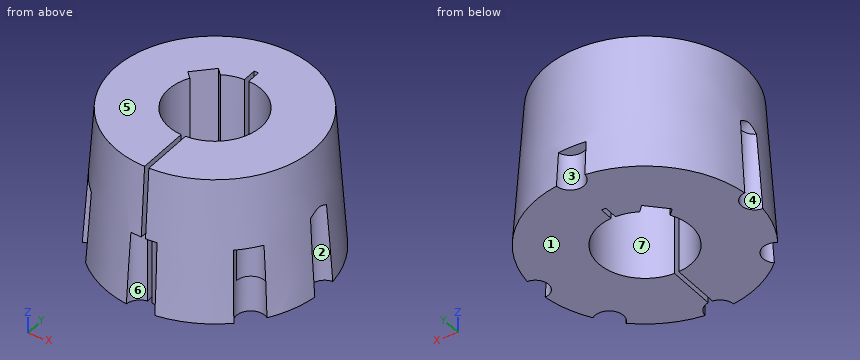
from build123d import *

# Parameters (mm, degrees)
CIRPATTERN1_COUNT       = 2
SKETCH7_R               = 10
CUT_EXTRUDE1_DEPTH      = 25
CIRPATTERN2_COUNT       = 2
CIRPATTERN2_ANGLE       = 130
SKETCH8_R               = 10
CUT_EXTRUDE2_DEPTH      = 50
CIRPATTERN3_COUNT       = 2
CIRPATTERN3_ANGLE       = 50
CUT_EXTRUDE3_DEPTH      = 1022.226122136
CUT_EXTRUDE3_DEPTH_BACK = 1022.226122136
SKETCH9_W               = 3
SKETCH9_H               = 87.216165293
CUT_EXTRUDE4_DEPTH      = 1022.226122136
CUT_EXTRUDE4_DEPTH_BACK = 1022.226122136
SKETCH12_R              = 10
CUT_EXTRUDE6_DEPTH      = 50
CUT_EXTRUDE7_DEPTH      = 1022.226122136
CUT_EXTRUDE7_DEPTH_BACK = 1022.226122136


with BuildPart() as part:
    # Sketch1 → Revolve1 (revolve)
    with BuildSketch(Plane(origin=(0, 0, 0), x_dir=(0, 0, -1), z_dir=(1, 0, 0)), mode=Mode.PRIVATE) as revolve1_sk:
        Polygon((627.254740219, 1014.21395543), (528.454740219, 1007.30518641), (528.454740219, 969.80518641), (532.567237031, 969.80518641), (611.238311694, 969.80518641), (627.254740219, 969.80518641), align=None)
    revolve(revolve1_sk.sketch.rotate(Axis((0, 937.30518641, -528.454740219), (0, 0, -1)), 90), axis=Axis((0, 937.30518641, -528.454740219), (0, 0, -1)))

    # Sketch6 → M20x1.5 Tapped Hole1 (revolve, cut)
    with BuildSketch(Plane(origin=(-76.90876902, 937.30518641, -627.254740219), x_dir=(0, 1, 0), z_dir=(1, 0, 0))):
        Polygon((0, 0), (0, 60.057960726), (9.25, 54.5), (9.25, 0), align=None)
    m20x1_5_tapped_hole1 = revolve(axis=Axis((-76.90876902, 937.30518641, -633.604740219), (0, 0, 1)), mode=Mode.SUBTRACT)

    # CirPattern1: M20x1.5 Tapped Hole1 ×2 about axis
    cirpattern1_axis = Axis((0, 937.30518641, 0), (0, 0, 1))
    for i in range(1, CIRPATTERN1_COUNT):
        add(m20x1_5_tapped_hole1.rotate(cirpattern1_axis, i * 360 / CIRPATTERN1_COUNT), mode=Mode.SUBTRACT)

    # Sketch7 → Cut-Extrude1 (cut)
    with BuildSketch(Plane(origin=(0, 0, -627.254740219), x_dir=(-1, 0, 0), z_dir=(0, 0, -1))):
        with Locations((0, 1014.21395543)):
            Circle(SKETCH7_R)
    cut_extrude1 = extrude(amount=-CUT_EXTRUDE1_DEPTH, mode=Mode.SUBTRACT)

    # CirPattern2: Cut-Extrude1 ×2 about axis
    cirpattern2_axis = Axis((0, 937.30518641, -627.254740219), (0, 0, -1))
    for i in range(1, CIRPATTERN2_COUNT):
        add(cut_extrude1.rotate(cirpattern2_axis, i * CIRPATTERN2_ANGLE / (CIRPATTERN2_COUNT - 1)), mode=Mode.SUBTRACT)

    # Sketch8 → Cut-Extrude2 (cut)
    with BuildSketch(Plane(origin=(0, 0, -627.254740219), x_dir=(-1, 0, 0), z_dir=(0, 0, -1))):
        with Locations((0, 860.39641739)):
            Circle(SKETCH8_R)
    cut_extrude2 = extrude(amount=-CUT_EXTRUDE2_DEPTH, mode=Mode.SUBTRACT)

    # CirPattern3: Cut-Extrude2 ×2 about axis
    cirpattern3_axis = Axis((0, 937.30518641, -627.254740219), (0, 0, -1))
    for i in range(1, CIRPATTERN3_COUNT):
        add(cut_extrude2.rotate(cirpattern3_axis, i * CIRPATTERN3_ANGLE / (CIRPATTERN3_COUNT - 1)), mode=Mode.SUBTRACT)

    # Sketch9 → Cut-Extrude3 (cut, two sides: drawn at the far end of the back side and taken through both)
    with BuildSketch(Plane(origin=(0, 0, -627.254740219), x_dir=(-1, 0, 0), z_dir=(0, 0, -1)).offset(-CUT_EXTRUDE3_DEPTH_BACK)):
        with Locations((0, 893.697103764)):
            Rectangle(SKETCH9_W, SKETCH9_H)
    extrude(amount=CUT_EXTRUDE3_DEPTH + CUT_EXTRUDE3_DEPTH_BACK, mode=Mode.SUBTRACT)

    # Sketch10 → Cut-Extrude4 (cut, two sides: drawn at the far end of the back side and taken through both)
    with BuildSketch(Plane(origin=(0, 0, -627.254740219), x_dir=(-1, 0, 0), z_dir=(0, 0, -1)).offset(-CUT_EXTRUDE4_DEPTH_BACK)):
        Polygon((1.5, 957.30518641), (1.5, 979.639325832), (-1.5, 979.639325832), (-1.5, 957.30518641), (-1.5, 953.730478501), (1.5, 953.730478501), align=None)
    extrude(amount=CUT_EXTRUDE4_DEPTH + CUT_EXTRUDE4_DEPTH_BACK, mode=Mode.SUBTRACT)

    # Sketch12 → Cut-Extrude6 (cut)
    with BuildSketch(Plane(origin=(0, 0, -627.254740219), x_dir=(-1, 0, 0), z_dir=(0, 0, -1))):
        with Locations((-58.915535135, 887.869182608)):
            Circle(SKETCH12_R)
    extrude(amount=-CUT_EXTRUDE6_DEPTH, mode=Mode.SUBTRACT)

    # Sketch13 → Cut-Extrude7 (cut, two sides: drawn at the far end of the back side and taken through both)
    with BuildSketch(Plane(origin=(0, 0, -627.254740219), x_dir=(-1, 0, 0), z_dir=(0, 0, -1)).offset(-CUT_EXTRUDE7_DEPTH_BACK)):
        Polygon((13.05698563, 963.090094101), (25.784907691, 950.36217204), (32.855975503, 957.433239852), (20.128053442, 970.161161913), align=None)
    extrude(amount=CUT_EXTRUDE7_DEPTH + CUT_EXTRUDE7_DEPTH_BACK, mode=Mode.SUBTRACT)


solid = part.part
Read the model definition and answer for the solid it produces. Units are mm, in the model's axes. Face numbers are marked on the shaded views. A direction names the side the tool comes from. Coordinates: 2 decimals unless noted, no trailing zeros. Loops run counter-clockwise (first coordinate to the right, second up) from the corner with the lowest first, then second, coordinate; pieces in that order, holes last.
Q1. Which of the six approach directions +Z, -Z, +X, -X, +Y, -Y give full straight-line access (tool end or side, diameter ignored) to the marked faces 5, 6 and 7?
Q2. Each of these flat-tipped pins is pushed along its axis until it touches: pin 1 Ø2 at (x, z) = (-41, -570) entering from +Y; pin 2 Ø1.9 at (x, y) = (5.5, 868.5) entering from -Z; pin 3 Ø4 at (x, z) = (-12.5, -582) entering from +Y; pin 4 Ø3 at (y, z) = (986.5, -581) entering from -X. Where does it stop, or does it pass through?
Q3. The part is cut by section A-A on z = -582.5. Write down the section's boundary in (x, y).
Q4. The mould has two halves that part along X. Classify the marked faces 1, 2, 3 and 4: +X half, -X half, draft (parallel to the pull), parting line (faces both ways), or undercut.
Q5. Consider probe 1 along Y at (x, z) = (-29, -556); probe 2 along X at (y, z) = (937.5, -590.5); probe 3 along Y at (x, z) = (-15.5, -599). Determine where each line is inside the solid, lowest interval first.
Results below:
1. face 5: +Z, +X, -X, +Y, -Y
1. face 6: -Z, -Y
1. face 7: +Z, -Z
2. pin 1: stops at y = 998.26
2. pin 2: stops at z = -627.25
2. pin 3: stops at y = 1010.33
2. pin 4: stops at x = -56.16
3. outline: (-73.29, 928.79) arc R73.78 ccw to (-62.04, 897.37) arc R10 cw to (-50.1, 883.15) arc R73.78 ccw to (-9.28, 864.11) arc R10 cw to (-1.5, 870.28) - (-1.5, 904.84) arc R32.5 cw to (-28.45, 953.02) - (-32.86, 957.43) - (-20.13, 970.16) - (-15.72, 965.75) arc R32.5 cw to (-1.5, 969.77) - (-1.5, 979.64) - (1.5, 979.64) - (1.5, 969.77) arc R32.5 cw to (1.5, 904.84) - (1.5, 870.28) arc R10 cw to (9.28, 864.11) arc R73.78 ccw to (50.1, 883.15) arc R10 cw to (62.04, 897.37) arc R73.78 ccw to (73.29, 928.79) arc R9.25 cw to (73.29, 945.82) arc R73.78 ccw to (-73.29, 945.82) arc R9.25 cw to start
4. face 1: draft
4. face 2: +X half
4. face 3: undercut
4. face 4: -X half
5. probe 1: y = 871.48 to 922.63, 951.98 to 953.58, 961.29 to 1003.13
5. probe 2: x = -67.66 to -32.5, 32.5 to 67.66
5. probe 3: y = 863.99 to 908.74, 965.87 to 1010.62
